```python
from build123d import *

# Parameters (mm, degrees)
SKETCH_1_R               = 1.5
EXTRUDE_1_DEPTH          = 66.5
CUT_EXTRUDE_1_DEPTH      = 72.43397301
CUT_EXTRUDE_1_DEPTH_BACK = 29.5
CUT_EXTRUDE_2_DEPTH      = 50
SKETCH_1_4_R             = 8.25
CUT_EXTRUDE_3_DEPTH      = 60
EXTRUDE_2_DEPTH          = 2.25


with BuildPart() as part:
    # Sketch 1 → Extrude 1 (new body)
    with BuildSketch(Plane.XY):
        with BuildLine():
            Line((-16.75, -10.928746497), (-7.681906247, 15.784996271))
            ThreePointArc((-7.681906247, 15.784996271), (-5.835532469, 18.470596932), (-2.857607815, 19.794799256))
            ThreePointArc((-2.857607815, 19.794799256), (0, 20), (2.857607815, 19.794799256))
            ThreePointArc((2.857607815, 19.794799256), (5.835532469, 18.470596932), (7.681906247, 15.784996271))
            Line((7.681906247, 15.784996271), (16.75, -10.928746497))
            ThreePointArc((16.75, -10.928746497), (0, -20), (-16.75, -10.928746497))
        make_face()
        with Locations((0, 16)):
            Circle(SKETCH_1_R, mode=Mode.SUBTRACT)
    extrude(amount=EXTRUDE_1_DEPTH)

    # Sketch 2 → Cut-Extrude 1 (cut, two sides: drawn at the far end of the back side and taken through both)
    with BuildSketch(Plane.XY.offset(66.5).offset(-CUT_EXTRUDE_1_DEPTH_BACK)):
        with BuildLine():
            Line((3.464101615, 14), (5.975770193, 18.350337589))
            ThreePointArc((5.975770193, 18.350337589), (4.522314785, 19.300583014), (2.857607815, 19.794799256))
            ThreePointArc((2.857607815, 19.794799256), (0, 20), (-2.857607815, 19.794799256))
            ThreePointArc((-2.857607815, 19.794799256), (-3.435719859, 19.682133501), (-4, 19.513328789))
            Line((-4, 19.513328789), (-4, 16))
            ThreePointArc((-4, 16), (-1.03527618, 12.136296695), (3.464101615, 14))
        make_face()
    extrude(amount=CUT_EXTRUDE_1_DEPTH + CUT_EXTRUDE_1_DEPTH_BACK, mode=Mode.SUBTRACT)

    # Sketch 1_3 → Cut-Extrude 2 (cut)
    with BuildSketch(Plane.XY):
        with BuildLine():
            Line((-10, 0), (-10, -17.320508076))
            ThreePointArc((-10, -17.320508076), (4.648040342, -19.452396279), (16.75, -10.928746497))
            Line((16.75, -10.928746497), (9.645647869, 10))
            Line((9.645647869, 10), (0, 10))
            ThreePointArc((0, 10), (-7.071067812, 7.071067812), (-10, 0))
        make_face()
    extrude(amount=CUT_EXTRUDE_2_DEPTH, mode=Mode.SUBTRACT)

    # Sketch 1_4 → Cut-Extrude 3 (cut)
    with BuildSketch(Plane.XY):
        Circle(SKETCH_1_4_R)
    extrude(amount=CUT_EXTRUDE_3_DEPTH, mode=Mode.SUBTRACT)

    # Sketch 3 → Extrude 2 (add, symmetric)
    with BuildSketch(Plane(origin=(0, 0, 0), x_dir=(0, 0, -1), z_dir=(1, 0, 0))):
        Polygon((-66.5, 9.75), (-66.5, -2.75), (-74.5, -2.75), align=None)
    extrude(amount=EXTRUDE_2_DEPTH, both=True)


solid = part.part
```
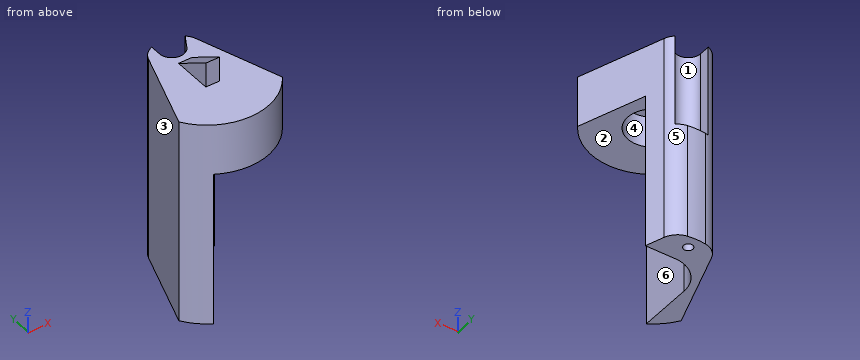
CAD build for the part. Positions are in the model's coordinates, mm. Face numbers are marked on the shaded views. A direction names the side the tool comes from. Coordinates: 2 decimals unless noted, no trailing zeros. Write each loop counter-clockwise with the first axis right and the second up, starting at its lowest first coordinate (ties: lowest second). Pieces come first, ordered by that corner, then holes.
(1) 3-axis set-ups, long thin cutter, end or side, ignore diameter. For the marked faces 5 and 6: which of +Z, -Z, +X, -X, +Y, -Y reach the whole face in a straight line?
(2) Drill centre lines: probe 1 along Y at (x, z) = (0, 19); probe 2 along Y at (x, z) = (0, 52); probe 3 along Z at (x, y) = (7, 8). Where is each one in solid material? Low to high.
(3) Cut at D-D, the plane y = -12. List the corners of the cut face in (x, z).
(4) Cut at C-C, the plane y = -4. List the corners of the cut face in (x, z), and give its area (3 significant figures).
(5) Two-plate mould, pull along X, no slides. Class the marked faces 1, 2, 3 and 4: +X half, -X half, draft (parallel to the pull), parting line (faces both ways), or undercut.
(6) Flat gauge pins, fed straight in: pin 1 (12 mm diameter, centred on y = -13, z = 36.5, fed in from +X); pin 2 (2 mm diameter, centred on x = 6.5, z = 27.5, fed in from -Y); pin 3 (2.5 mm diameter, centred on y = 5, z = 70.5, fed in from -X); pin 4 (2.5 mm diameter, centred on x = 0, y = 16, fed in from +Z). Where does each tip first touch, or does it go through?
Geometry says:
1. face 5: +Z, -Z, +X, +Y
1. face 6: -Z, +X, -Y
2. probe 1: y = 10 to 14.5, 17.5 to 20
2. probe 2: y = -20 to -8.25, 8.25 to 12
2. probe 3: z = 50 to 66.5
3. outline: (-16, 0) - (-10, 0) - (-10, 50) - (16, 50) - (16, 66.5) - (-16, 66.5) - close
4. outline: (-14.4, 0) - (-10, 0) - (-10, 50) - (-7.22, 50) - (-7.22, 60) - (7.22, 60) - (7.22, 50) - (14.4, 50) - (14.4, 66.5) - (-14.4, 66.5) - close
4. area: 551 mm2
5. face 1: undercut
5. face 2: draft
5. face 3: -X half
5. face 4: undercut
6. pin 1: stops at x = -10
6. pin 2: stops at y = 10
6. pin 3: stops at x = -2.25
6. pin 4: passes through
